Source: CAD feature listing. Evaluate the final solid. Frame: model axes, mm. Round coordinates to 2 decimals unless told otherwise and drop trailing zeros. Order: outer loops, then holes, each group sorted by start corner. A loop starts at its lowest first (then second) coordinate and runs counter-clockwise, first axis right, second up. Notation, with made-up numbers: M 1.25,-7.5 L 29.25,-7.5 A13 ccw 29.25,10.5 Z; hole C 42,85 d11. An arc over 180 degrees is marked long. Use one line per item in the form item = value. Start each with the question number.
Q1. Section A-A (x = 125). Return the cut outline in (y, z), plus the area to 3 significant figures.
Q2. Section B-B (z = -129). Return the cut outline in (x, y), plus the area to 3 significant figures.
Q3. Section C-C (y = 1.1). Give the number of separate pieces and of enclosed holes in the cut face, plus the area to 3 significant figures.
Q4. Contact query for a flat-ended pin moving along its axis: pin 1 (1.4 mm diameter, centred on x = 101.6, z = -25.4, fed in from -Y). Output: stop coordinate, or through.
Q5. Material intervals for probe 1 along Z at (x, y) = (63.5, 1.2); probe 2 along X at (y, z) = (2.5, -187); probe 3 along X at (y, z) = (1.55, -311.15), sorted ascending.
from build123d import *

# Parameters (mm, degrees)
SKETCH1_W                 = 203.2
SKETCH1_H                 = 431.8
BOSS_EXTRUDE1_DEPTH       = 5.8
M3X0_5_TAPPED_HOLE2_D     = 2.5
M3X0_5_TAPPED_HOLE2_DEPTH = 7.5
M3X0_5_TAPPED_HOLE2_TIP   = 0.751075774
SKETCH7_W                 = 63.5
SKETCH7_H                 = 355.6
CUT_EXTRUDE2_DEPTH        = 478.257917692
FILLET1_R                 = 25.4
M3X0_5_TAPPED_HOLE1_D     = 2.5
M3X0_5_TAPPED_HOLE1_DEPTH = 7.5
M3X0_5_TAPPED_HOLE1_TIP   = 0.751075774
SKETCH10_R                = 0.79375
CUT_EXTRUDE3_DEPTH        = 478.257917692


with BuildPart() as part:
    # Sketch1 → Boss-Extrude1 (new body)
    with BuildSketch(Plane(origin=(0, 0, 0), x_dir=(1, 0, 0), z_dir=(0, 1, 0))):
        with Locations((101.6, 215.9)):
            Rectangle(SKETCH1_W, SKETCH1_H)
    extrude(amount=BOSS_EXTRUDE1_DEPTH)

    # M3x0.5 Tapped Hole2
    with Locations(Plane(origin=(0, 5.8, 0), x_dir=(-1, 0, 0), z_dir=(0, 1, 0))):
        with Locations((-63.5, -419.1), (-139.7, -419.1), (-63.5, -215.9), (-139.7, -215.9), (-63.5, -12.7), (-139.7, -12.7)):
            Hole(M3X0_5_TAPPED_HOLE2_D / 2, depth=M3X0_5_TAPPED_HOLE2_DEPTH)
            with Locations((0, 0, -(M3X0_5_TAPPED_HOLE2_DEPTH + M3X0_5_TAPPED_HOLE2_TIP / 2))):  # 118° drill point
                Cone(0, M3X0_5_TAPPED_HOLE2_D / 2, M3X0_5_TAPPED_HOLE2_TIP, mode=Mode.SUBTRACT)

    # Sketch7 → Cut-Extrude2 (cut, through all)
    with BuildSketch(Plane(origin=(0, 5.8, 0), x_dir=(1, 0, 0), z_dir=(0, 1, 0))):
        with Locations((101.6, 215.9)):
            Rectangle(SKETCH7_W, SKETCH7_H)
    extrude(amount=-CUT_EXTRUDE2_DEPTH, mode=Mode.SUBTRACT)

    # Fillet1
    fillet1_edges = [part.edges().sort_by_distance(p)[0] for p in [
        (0, 2.9, -431.8),
        (203.2, 2.9, -431.8),
        (203.2, 2.9, 0),
        (0, 2.9, 0),
    ]]
    fillet(fillet1_edges, radius=FILLET1_R)

    # M3x0.5 Tapped Hole1
    with Locations(Plane(origin=(0, 5.8, 0), x_dir=(-1, 0, 0), z_dir=(0, 1, 0))):
        with Locations((-190.5, -406.4), (-190.5, -25.4), (-12.7, -25.4), (-12.7, -406.4), (-190.5, -215.9), (-12.7, -215.9)):
            Hole(M3X0_5_TAPPED_HOLE1_D / 2, depth=M3X0_5_TAPPED_HOLE1_DEPTH)
            with Locations((0, 0, -(M3X0_5_TAPPED_HOLE1_DEPTH + M3X0_5_TAPPED_HOLE1_TIP / 2))):  # 118° drill point
                Cone(0, M3X0_5_TAPPED_HOLE1_D / 2, M3X0_5_TAPPED_HOLE1_TIP, mode=Mode.SUBTRACT)

    # Sketch10 → Cut-Extrude3 (cut, through all)
    with BuildSketch(Plane(origin=(0, 5.8, 0), x_dir=(1, 0, 0), z_dir=(0, 1, 0))):
        with Locations(Location((12.7, 311.15, 0), (0, 0, 270))):
            Circle(SKETCH10_R)
        with Locations(Location((190.5, 311.15, 0), (0, 0, 270))):
            Circle(SKETCH10_R)
        with Locations(Location((101.6, 406.4, 0), (0, 0, 270))):
            Circle(SKETCH10_R)
        with Locations(Location((101.6, 25.4, 0), (0, 0, 90))):
            Circle(SKETCH10_R)
        with Locations(Location((190.5, 120.65, 0), (0, 0, 90))):
            Circle(SKETCH10_R)
        with Locations(Location((12.7, 120.65, 0), (0, 0, 90))):
            Circle(SKETCH10_R)
    extrude(amount=-CUT_EXTRUDE3_DEPTH, mode=Mode.SUBTRACT)


solid = part.part
Results list:
q1.outline = M 0,-431.8 L 5.8,-431.8 L 5.8,-393.7 L 0,-393.7 Z; M 0,-38.1 L 5.8,-38.1 L 5.8,0 L 0,0 Z
q1.area = 442 mm2
q2.outline = M 0,0 L 69.85,0 L 69.85,5.8 L 0,5.8 Z; M 133.35,0 L 203.2,0 L 203.2,5.8 L 133.35,5.8 Z
q2.area = 810 mm2
q3.separate_pieces = 1
q3.enclosed_holes = 19
q3.area = 64,500 mm2
q4.pin_1 = through
q5.probe_1 = -431.8 to -420.35, -417.85 to -217.15, -214.65 to -13.95, -11.45 to 0
q5.probe_2 = 0 to 69.85, 133.35 to 203.2
q5.probe_3 = 0 to 11.91, 13.49 to 69.85, 133.35 to 189.71, 191.29 to 203.2
